from build123d import *

# Parameters (mm, degrees)
F1_DEPTH = 1000
F2_R     = 4
F3_R     = 2
F5_D     = 5


with BuildPart() as f1:
    # F0 (on Front) → F1 (new body)
    with BuildSketch(Plane.XZ):
        Polygon((-60, 20), (0, 0), (60, 20), (60, 70), (58, 70), (58, 21.441518), (0, 2.108185), (-58, 21.441518), (-58, 70), (-60, 70), align=None)
    extrude(amount=F1_DEPTH)

    # F2
    f2_edges = [f1.edges().sort_by_distance(p)[0] for p in [
        (60, -500, 20),
        (0, -500, 0),
        (-60, -500, 20),
    ]]
    fillet(f2_edges, radius=F2_R)

    # F3
    f3_edges = [f1.edges().sort_by_distance(p)[0] for p in [
        (-58, -500, 21.441518),
        (0, -500, 2.108185),
        (58, -500, 21.441518),
    ]]
    fillet(f3_edges, radius=F3_R)

    # F5 (through all)
    with Locations(Plane(origin=(-60, 0, 0), x_dir=(0, -1, 0), z_dir=(-1, 0, 0))):
        with Locations((100, 50), (130, 50), (870, 50), (900, 50)):
            Hole(F5_D / 2)


solid = f1.part
The listing builds one solid part. Answer for the finished solid, in the listing's coordinates (mm). A direction names the side the tool comes from. Round coordinates to 2 decimals unless told otherwise and drop trailing zeros. Write each loop counter-clockwise with the first axis right and the second up, starting at its lowest first coordinate (ties: lowest second). Pieces come first, ordered by that corner, then holes. Notation, with made-up numbers: (73, 26) - (94, 26) arc R28 cw to (94, 54) - close; hole circle Ø9 at (-6, 34.25). An arc over 180 degrees is marked (long way). Use one line per item in the form item = value. Start each with the question number.
Item 1: A cutting plane is placed at A-A (z = 33). Write down the section's boundary in (x, y), plus the area to 3 significant figures.
Item 2: Determine the mould class of faces 3 (the flat face through (58, -493, 47)), 4 (the flat face through (-60, -493, 47)), 5 (the flat face through (-31, 0, 12)) for opening direction X: +X half, -X half, draft (parallel to the pull), parting line (faces both ways), or undercut.
Item 3: A cutting plane is placed at C-C (x = -37.5). Write down the section's boundary in (y, z), plus the area to 3 significant figures.
Item 4: A cutting plane is placed at B-B (y = -237). Write down the section's boundary in (x, z).
Item 5: Flat-ended cylindrical pins translate along their axes: pin 1 Ø3 at (x, y) = (25.5, -560.5) entering from +Z; pin 2 Ø1 at (x, y) = (10.5, -154.5) entering from +Z; pin 3 Ø5 at (x, y) = (19.5, -169.5) entering from -Z. Find the tip coordinate at first contact, or state that the pin passes through.
Item 6: A tool of negligible diameter and unlimited length cuts with its end or side. For faces 1 (the flat face through (60, -493, 46)), 2 (the flat face through (29.02, -493, 11.78)), from which of +Z, -Z, +X, -X, +Y, -Y can it reach the whole face along a straight path? Write none if from no direction.
Item 7: Find the intervals of material crossed by line 1 (X direction, y = -562, z = 44); line 2 (Z direction, x = 59.2, y = -870); line 3 (Z direction, x = -58.5, y = -130), in increasing order. Write a range as [from, to].
The answers:
q1.outline = (-60, -1000) - (-58, -1000) - (-58, 0) - (-60, 0) - close; (58, -1000) - (60, -1000) - (60, 0) - (58, 0) - close
q1.area = 4,000 mm^2
q2.face_3 = undercut
q2.face_4 = -X half
q2.face_5 = draft
q3.outline = (-1000, 12.5) - (0, 12.5) - (0, 14.61) - (-1000, 14.61) - close
q3.area = 2,110 mm^2
q4.outline = (-60, 22.88) arc R4 ccw to (-57.26, 19.09) - (-1.26, 0.42) arc R4 ccw to (1.26, 0.42) - (57.26, 19.09) arc R4 ccw to (60, 22.88) - (60, 70) - (58, 70) - (58, 22.88) arc R2 cw to (56.63, 20.99) - (0.63, 2.32) arc R2 cw to (-0.63, 2.32) - (-56.63, 20.99) arc R2 cw to (-58, 22.88) - (-58, 70) - (-60, 70) - close
q5.pin_1 = 11.11
q5.pin_2 = 5.77
q5.pin_3 = 5.67
q6.face_1 = +Z, -Z, +X, +Y, -Y
q6.face_2 = +Z, +Y, -Y
q7.line_1 = [-60, -58], [58, 60]
q7.line_2 = [20.48, 47.5], [52.5, 70]
q7.line_3 = [19.76, 47.5], [52.5, 70]
